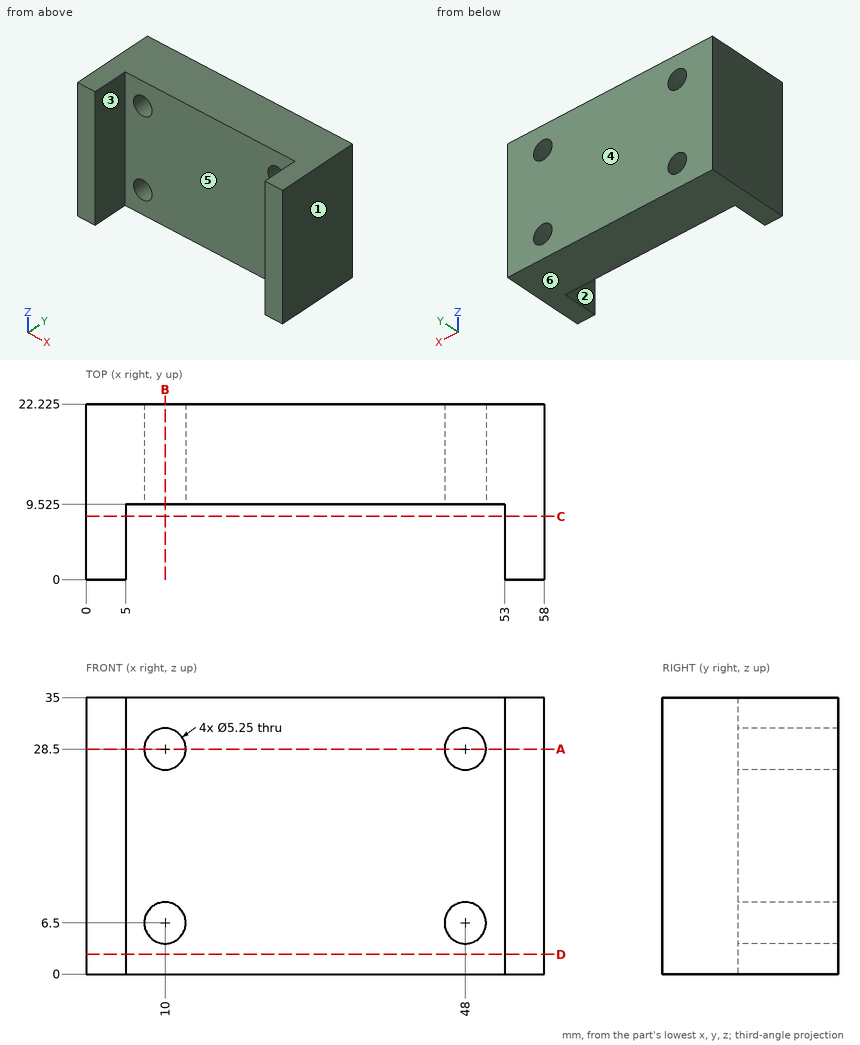
Geometry: see drawing. Coordinates: mm, zero at the bounding-box minimum. A direction names the side the tool comes from. Give positions to 0.01 mm unless a question says otherwise; leave off trailing zeros. Order: outer loops, then holes, each group sorted by start corner. A loop starts at its lowest first (then second) coordinate and runs counter-clockwise, first axis right, second up. Notation, with made-up numbers: M 23.5,52.5 L 78.5,52.5 A22 cw 78.5,60.5 Z; hole C -18.5,-3.5 d6. An arc over 180 degrees is marked long. Answer as a JSON object with one key per item and string values.
1. Cut plane D-D, the plane z = 2.5. Output: boundary loops of the cut face in (x, y) (3 decimals).
Result sheet:
{"outline": "M 0,0 L 5,0 L 5,9.525 L 53,9.525 L 53,0 L 58,0 L 58,22.225 L 0,22.225 Z"}
2. Cut plane B-B, the plane x = 10. Output: boundary loops of the cut face in (y, z) (3 decimals).
Result sheet:
{"outline": "M 9.525,0 L 22.225,0 L 22.225,3.875 L 9.525,3.875 Z; M 9.525,9.125 L 22.225,9.125 L 22.225,25.875 L 9.525,25.875 Z; M 9.525,31.125 L 22.225,31.125 L 22.225,35 L 9.525,35 Z"}
3. Ray query, line 1 (X direction, y = 13.75, z = 6.5) (3 decimals); line 2 (Z direction, x = 10, y = 14) (3 decimals); line 3 (X direction, y = 1.5, z = 26). Return the intervals inside material, ascending. Write a range as [from, to].
Result sheet:
{"line 1": "[0, 7.375], [12.625, 45.375], [50.625, 58]", "line 2": "[0, 3.875], [9.125, 25.875], [31.125, 35]", "line 3": "[0, 5], [53, 58]"}
4. Cut plane A-A, the plane z = 28.5. Output: boundary loops of the cut face in (x, y) (3 decimals), and give its area (4 significant figures).
Result sheet:
{"outline": "M 0,0 L 5,0 L 5,9.525 L 7.375,9.525 L 7.375,22.225 L 0,22.225 Z; M 12.625,9.525 L 45.375,9.525 L 45.375,22.225 L 12.625,22.225 Z; M 50.625,9.525 L 53,9.525 L 53,0 L 58,0 L 58,22.225 L 50.625,22.225 Z", "area": "698.5 mm²"}
5. First-contact query: P1, Ø1.5, axis at x = 6, z = 6, coming from the -Y side (3 decimals); P2, Ø6, axis at x = 10, z = 28.5, coming from the +Y side (3 decimals). Flat tips, straight axial feed; report the tip coordinate or a pass-through.
Result sheet:
{"P1": "y = 9.525", "P2": "y = 22.225"}
6. Cut plane C-C, the plane y = 8. Output: boundary loops of the cut face in (x, z).
Result sheet:
{"outline": "M 0,0 L 5,0 L 5,35 L 0,35 Z; M 53,0 L 58,0 L 58,35 L 53,35 Z"}
7. Reachability of the marked faces 5 and 6 from +Z, -Z, +X, -X, +Y, -Y: full face, straight path, thin tool, end or side. Return the list, or none.
Result sheet:
{"face 5": "+Z, -Z, -Y", "face 6": "-Z, +X, -X, +Y, -Y"}
8. Pull-direction query (X, two-part tool) for the marked faces 1, 2, 3 and 4; classes: +X half, -X half, draft (parallel to the pull), parting line (faces both ways), or undercut.
Result sheet:
{"face 1": "+X half", "face 2": "undercut", "face 3": "undercut", "face 4": "draft"}
